```python
from build123d import *

# Parameters (mm, degrees)
F0_W     = 18
F0_H     = 11
F0_R     = 3
F1_DEPTH = 5
F2_W     = 18
F2_H     = 11
F3_DEPTH = 2
F4_R     = 3
F5_R     = 1.725
F6_DEPTH = 25


with BuildPart() as f1:
    # F0 (on Top) → F1 (new body)
    with BuildSketch(Plane.XY):
        Rectangle(F0_W, F0_H)
        with Locations((-4, 0)):
            Circle(F0_R, mode=Mode.SUBTRACT)
        with Locations((4, 0)):
            Circle(F0_R, mode=Mode.SUBTRACT)
    extrude(amount=F1_DEPTH)

    # F2 (on face) → F3 (join)
    with BuildSketch(Plane.XY.offset(5)):
        Rectangle(F2_W, F2_H)
    extrude(amount=F3_DEPTH)

    # F4
    f4_edges = [f1.edges().sort_by_distance(p)[0] for p in [
        (-9, 5.5, 3.5),
        (-9, -5.5, 3.5),
        (9, -5.5, 3.5),
        (9, 5.5, 3.5),
        (0, 5.5, 7),
        (0, -5.5, 7),
        (-9, 0, 7),
        (9, 0, 7),
    ]]
    fillet(f4_edges, radius=F4_R)

    # F5 (on face) → F6 (cut)
    with BuildSketch(Plane(origin=(0, 0, 5), x_dir=(1, 0, 0), z_dir=(0, 0, -1))):
        with Locations((-4, 0)):
            Circle(F5_R)
        with Locations((4, 0)):
            Circle(F5_R)
    extrude(amount=-F6_DEPTH, mode=Mode.SUBTRACT)


solid = f1.part
```
CAD build for the part. Positions are in the model's coordinates, mm. A direction names the side the tool comes from. Coordinates: 2 decimals unless noted, no trailing zeros. Write each loop counter-clockwise with the first axis right and the second up, starting at its lowest first coordinate (ties: lowest second). Pieces come first, ordered by that corner, then holes. Notation, with made-up numbers: (-33, -7) -> (5, -7) arc R38 cw to (5, 32) -> close; hole circle Ø1 at (-24.75, 72.5). An arc over 180 degrees is marked (long way). Return JSON: item names as keys, results as strings. Group by question number.
Q1. Which spindle directions (+Z, -Z, +X, -X, +Y, -Y) get a long thin tool onto all of the face, cutting with end or side? Do faces 4 (the face through (-5.27, -1.17, 5.99)), 5 (the face through (4, -2, 5)). Say none if no direction does.
Q2. Cut at B-B, the plane y = 0. Give the cut face in (x, z) (3 decimals), then the cut area to 3 significant figures.
Q3. Pull direction Y, two halves, no side cores. Call faces 1 (the face through (1, 0, 2)), 2 (the face through (9, 0, 2)), 3 (the face through (-8.14, 4.6, 1.97)): released by +Y, released by -Y, zero draft, split by the parting line, or undercut.
Q4. Drill centre lines: line 1 (Y direction, x = 4, z = 2.9); line 2 (X direction, y = 1.75, z = 1.5); line 3 (X direction, y = 0, z = 5.75) (3 decimals). Where is each one in solid material? Low to high.
Q5. Cut at A-A, the plane x = 4. Give the cut face in (y, z) (3 decimals), then the cut area to 3 significant figures.
Q6. Cut at C-C, the plane z = 1.5. Give the cut face in (x, y).
Q7. Cut at D-D, the plane x = -3.5. Give the cut face in (y, z).
Returned:
{
 "1": {"face 4": "+Z, -Z", "face 5": "-Z"},
 "2": {"outline": "(-9, 0) -> (-7, 0) -> (-7, 5) -> (-5.725, 5) -> (-5.725, 7) -> (-6, 7) arc R3 ccw to (-9, 4) -> close; (-2.275, 5) -> (-1, 5) -> (-1, 0) -> (1, 0) -> (1, 5) -> (2.275, 5) -> (2.275, 7) -> (-2.275, 7) -> close; (5.725, 5) -> (7, 5) -> (7, 0) -> (9, 0) -> (9, 4) arc R3 ccw to (6, 7) -> (5.725, 7) -> close", "area": "48.3 mm2"},
 "3": {"face 1": "undercut", "face 2": "zero draft", "face 3": "released by +Y"},
 "4": {"line 1": "y = -5.5 to -3, 3 to 5.5", "line 2": "x = -9 to -6.44, -1.56 to 1.56, 6.44 to 9", "line 3": "x = -8.437 to -5.725, -2.275 to 2.275, 5.725 to 8.437"},
 "5": {"outline": "(-5.5, 0) -> (-3, 0) -> (-3, 5) -> (-1.725, 5) -> (-1.725, 7) -> (-2.5, 7) arc R3 ccw to (-5.5, 4) -> close; (1.725, 5) -> (3, 5) -> (3, 0) -> (5.5, 0) -> (5.5, 4) arc R3 ccw to (2.5, 7) -> (1.725, 7) -> close", "area": "36.2 mm2"},
 "6": {"outline": "(-9, -2.5) arc R3 ccw to (-6, -5.5) -> (6, -5.5) arc R3 ccw to (9, -2.5) -> (9, 2.5) arc R3 ccw to (6, 5.5) -> (-6, 5.5) arc R3 ccw to (-9, 2.5) -> close; hole circle Ø6 at (-4, 0); hole circle Ø6 at (4, 0)"},
 "7": {"outline": "(-5.5, 0) -> (-2.96, 0) -> (-2.96, 5) -> (-1.65, 5) -> (-1.65, 7) -> (-2.5, 7) arc R3 ccw to (-5.5, 4) -> close; (1.65, 5) -> (2.96, 5) -> (2.96, 0) -> (5.5, 0) -> (5.5, 4) arc R3 ccw to (2.5, 7) -> (1.65, 7) -> close"}
}
